from build123d import *

# Parameters (mm, degrees)
SKETCH_W                        = 78
SKETCH_H                        = 68
PAD_DEPTH                       = 29
SKETCH001_W                     = 71
SKETCH001_H                     = 61
POCKET_DEPTH                    = 25
SKETCH002_R                     = 2.5
PAD001_DEPTH                    = 3
SKETCH002_MIRRORED_2_R          = 2.5
PAD001_MIRRORED_2_DEPTH         = 3
SKETCH003_R                     = 3.111428
POCKET001_DEPTH                 = 3
SKETCH004_R                     = 1.4
POCKET002_DEPTH                 = 4
SKETCH004_MIRRORED002_2_R       = 1.4
POCKET002_MIRRORED002_2_DEPTH   = 4
SKETCH005_R                     = 2.5
PAD002_DEPTH                    = 3
SKETCH006_R                     = 1.1
POCKET003_DEPTH                 = 3
SKETCH007_W                     = 9
SKETCH007_H                     = 5
POCKET004_DEPTH                 = 3.5
SKETCH008_W                     = 9
SKETCH008_H                     = 5
POCKET005_DEPTH                 = 3.5
SKETCH009_R                     = 3
POCKET006_DEPTH                 = 3.5
FILLET_R                        = 2
CHAMFER_SIZE                    = 1
CHAMFER001_SIZE                 = 3
SKETCH010_R                     = 2
POCKET007_DEPTH                 = 282.933548
SKETCH010_LINEARPATTERN_2_R     = 2
POCKET007_LINEARPATTERN_2_DEPTH = 282.933548
SKETCH010_LINEARPATTERN_3_R     = 2
POCKET007_LINEARPATTERN_3_DEPTH = 282.933548
SKETCH010_LINEARPATTERN_4_R     = 2
POCKET007_LINEARPATTERN_4_DEPTH = 282.933548
SKETCH010_LINEARPATTERN_5_R     = 2
POCKET007_LINEARPATTERN_5_DEPTH = 282.933548
SKETCH010_LINEARPATTERN_6_R     = 2
POCKET007_LINEARPATTERN_6_DEPTH = 282.933548
SKETCH010_LINEARPATTERN_7_R     = 2
POCKET007_LINEARPATTERN_7_DEPTH = 282.933548
SKETCH010_LINEARPATTERN_8_R     = 2
POCKET007_LINEARPATTERN_8_DEPTH = 282.933548
SKETCH010_LINEARPATTERN_9_R     = 2
POCKET007_LINEARPATTERN_9_DEPTH = 282.933548
LINEARPATTERN001_COUNT          = 3
LINEARPATTERN001_PITCH          = 5
SKETCH011_W                     = 75
SKETCH011_H                     = 65
POCKET008_DEPTH                 = 3
SKETCH012_R                     = 1.564418
PAD003_DEPTH                    = 1


with BuildPart() as part:
    # Sketch → Pad (new body)
    with BuildSketch(Plane.XY):
        with Locations((39, 34)):
            Rectangle(SKETCH_W, SKETCH_H)
    extrude(amount=PAD_DEPTH)

    # Sketch001 (on Face6 of Pad) → Pocket (cut)
    with BuildSketch(Plane.XY.offset(29)):
        with Locations((39, 34)):
            Rectangle(SKETCH001_W, SKETCH001_H)
    extrude(amount=-POCKET_DEPTH, mode=Mode.SUBTRACT)

    # Sketch002 (on Face11 of Pocket) → Pad001 (join)
    with BuildSketch(Plane.XY.offset(4)):
        with Locations((8.5, 60)):
            Circle(SKETCH002_R)
    pad001 = extrude(amount=PAD001_DEPTH)

    # Sketch002 Mirrored 2 → Pad001 Mirrored 2 (add)
    with BuildSketch(Plane(origin=(0, 68, 4), x_dir=(1, 0, 0), z_dir=(0, 0, -1))):
        with Locations((8.5, 60)):
            Circle(SKETCH002_MIRRORED_2_R)
    pad001_mirrored_2 = extrude(amount=-PAD001_MIRRORED_2_DEPTH)

    # Mirrored001: Pad001, Pad001 Mirrored 2 across Sketch002 Axis3
    add(pad001.mirror(Plane(origin=(39, 64.5, 4), x_dir=(0, 0, 1), z_dir=(1, 0, 0))))
    add(pad001_mirrored_2.mirror(Plane(origin=(39, 64.5, 4), x_dir=(0, 0, 1), z_dir=(1, 0, 0))))

    # Sketch003 (on Face17 of MultiTransform) → Pocket001 (cut)
    with BuildSketch(Plane.XY.offset(7)):
        with Locations((69.5, 8)):
            Circle(SKETCH003_R)
    extrude(amount=-POCKET001_DEPTH, mode=Mode.SUBTRACT)

    # Sketch004 (on Face18 of Pocket001) → Pocket002 (cut)
    with BuildSketch(Plane.XY.offset(7)):
        with Locations((8.5, 60)):
            Circle(SKETCH004_R)
    pocket002 = extrude(amount=-POCKET002_DEPTH, mode=Mode.SUBTRACT)

    # Sketch004 Mirrored002 2 → Pocket002 Mirrored002 2 (cut)
    with BuildSketch(Plane(origin=(78, 0, 7), x_dir=(-1, 0, 0), z_dir=(0, 0, -1))):
        with Locations((8.5, 60)):
            Circle(SKETCH004_MIRRORED002_2_R)
    pocket002_mirrored002_2 = extrude(amount=POCKET002_MIRRORED002_2_DEPTH, mode=Mode.SUBTRACT)

    # Mirrored003: Pocket002, Pocket002 Mirrored002 2 across Sketch004 Axis2
    add(pocket002.mirror(Plane(origin=(39, 34, 7), x_dir=(0, 0, 1), z_dir=(0, 1, 0))), mode=Mode.SUBTRACT)
    add(pocket002_mirrored002_2.mirror(Plane(origin=(39, 34, 7), x_dir=(0, 0, 1), z_dir=(0, 1, 0))), mode=Mode.SUBTRACT)

    # Sketch005 (on Face11 of MultiTransform001) → Pad002 (join)
    with BuildSketch(Plane.XY.offset(4)):
        with Locations((49.5, 18)):
            Circle(SKETCH005_R)
    extrude(amount=PAD002_DEPTH)

    # Sketch006 (on Face19 of Pad002) → Pocket003 (cut)
    with BuildSketch(Plane.XY.offset(7)):
        with Locations((69.5, 60)):
            Circle(SKETCH006_R)
    extrude(amount=-POCKET003_DEPTH, mode=Mode.SUBTRACT)

    # Sketch007 (on Face3 of Pocket003) → Pocket004 (cut)
    with BuildSketch(Plane.YZ.offset(78)):
        with Locations((9.9, 11)):
            Rectangle(SKETCH007_W, SKETCH007_H)
    extrude(amount=-POCKET004_DEPTH, mode=Mode.SUBTRACT)

    # Sketch008 (on Face2 of Pocket004) → Pocket005 (cut)
    with BuildSketch(Plane(origin=(0, 0, 0), x_dir=(0, -1, 0), z_dir=(-1, 0, 0))):
        with Locations((-15.4, 11)):
            Rectangle(SKETCH008_W, SKETCH008_H)
    extrude(amount=-POCKET005_DEPTH, mode=Mode.SUBTRACT)

    # Sketch009 (on Face2 of Pocket005) → Pocket006 (cut)
    with BuildSketch(Plane(origin=(0, 0, 0), x_dir=(0, -1, 0), z_dir=(-1, 0, 0))):
        with Locations((-46, 11)):
            Circle(SKETCH009_R)
    extrude(amount=-POCKET006_DEPTH, mode=Mode.SUBTRACT)

    # Fillet
    fillet_edges = [part.edges().sort_by_distance(p)[0] for p in [
        (39, 0, 0),
        (78, 34, 0),
        (39, 68, 0),
        (0, 34, 0),
        (78, 0, 14.5),
        (0, 68, 14.5),
        (78, 68, 14.5),
        (0, 0, 14.5),
    ]]
    fillet(fillet_edges, radius=FILLET_R)

    # Chamfer
    chamfer_edges = [part.edges().sort_by_distance(p)[0] for p in [
        (78, 9.9, 8.5),
        (78, 5.4, 11),
        (78, 9.9, 13.5),
        (78, 14.4, 11),
        (0, 15.4, 8.5),
        (0, 19.9, 11),
        (0, 15.4, 13.5),
        (0, 10.9, 11),
    ]]
    chamfer(chamfer_edges, length=CHAMFER_SIZE)

    # Chamfer001
    chamfer001_edges = [part.edges().sort_by_distance(p)[0] for p in [
        (0, 49, 11),
    ]]
    chamfer(chamfer001_edges, length=CHAMFER001_SIZE)

    # Sketch010 (on Face16 of Chamfer001) → Pocket007 (cut, through all)
    with BuildSketch(Plane.XZ):
        with Locations((7, 12.5)):
            Circle(SKETCH010_R)
    pocket007 = extrude(amount=-POCKET007_DEPTH, mode=Mode.SUBTRACT)

    # Sketch010 LinearPattern 2 → Pocket007 LinearPattern 2 (cut, through all)
    with BuildSketch(Plane(origin=(8, 0, 0), x_dir=(1, 0, 0), z_dir=(0, -1, 0))):
        with Locations((7, 12.5)):
            Circle(SKETCH010_LINEARPATTERN_2_R)
    pocket007_linearpattern_2 = extrude(amount=-POCKET007_LINEARPATTERN_2_DEPTH, mode=Mode.SUBTRACT)

    # Sketch010 LinearPattern 3 → Pocket007 LinearPattern 3 (cut, through all)
    with BuildSketch(Plane(origin=(16, 0, 0), x_dir=(1, 0, 0), z_dir=(0, -1, 0))):
        with Locations((7, 12.5)):
            Circle(SKETCH010_LINEARPATTERN_3_R)
    pocket007_linearpattern_3 = extrude(amount=-POCKET007_LINEARPATTERN_3_DEPTH, mode=Mode.SUBTRACT)

    # Sketch010 LinearPattern 4 → Pocket007 LinearPattern 4 (cut, through all)
    with BuildSketch(Plane(origin=(24, 0, 0), x_dir=(1, 0, 0), z_dir=(0, -1, 0))):
        with Locations((7, 12.5)):
            Circle(SKETCH010_LINEARPATTERN_4_R)
    pocket007_linearpattern_4 = extrude(amount=-POCKET007_LINEARPATTERN_4_DEPTH, mode=Mode.SUBTRACT)

    # Sketch010 LinearPattern 5 → Pocket007 LinearPattern 5 (cut, through all)
    with BuildSketch(Plane(origin=(32, 0, 0), x_dir=(1, 0, 0), z_dir=(0, -1, 0))):
        with Locations((7, 12.5)):
            Circle(SKETCH010_LINEARPATTERN_5_R)
    pocket007_linearpattern_5 = extrude(amount=-POCKET007_LINEARPATTERN_5_DEPTH, mode=Mode.SUBTRACT)

    # Sketch010 LinearPattern 6 → Pocket007 LinearPattern 6 (cut, through all)
    with BuildSketch(Plane(origin=(40, 0, 0), x_dir=(1, 0, 0), z_dir=(0, -1, 0))):
        with Locations((7, 12.5)):
            Circle(SKETCH010_LINEARPATTERN_6_R)
    pocket007_linearpattern_6 = extrude(amount=-POCKET007_LINEARPATTERN_6_DEPTH, mode=Mode.SUBTRACT)

    # Sketch010 LinearPattern 7 → Pocket007 LinearPattern 7 (cut, through all)
    with BuildSketch(Plane(origin=(48, 0, 0), x_dir=(1, 0, 0), z_dir=(0, -1, 0))):
        with Locations((7, 12.5)):
            Circle(SKETCH010_LINEARPATTERN_7_R)
    pocket007_linearpattern_7 = extrude(amount=-POCKET007_LINEARPATTERN_7_DEPTH, mode=Mode.SUBTRACT)

    # Sketch010 LinearPattern 8 → Pocket007 LinearPattern 8 (cut, through all)
    with BuildSketch(Plane(origin=(56, 0, 0), x_dir=(1, 0, 0), z_dir=(0, -1, 0))):
        with Locations((7, 12.5)):
            Circle(SKETCH010_LINEARPATTERN_8_R)
    pocket007_linearpattern_8 = extrude(amount=-POCKET007_LINEARPATTERN_8_DEPTH, mode=Mode.SUBTRACT)

    # Sketch010 LinearPattern 9 → Pocket007 LinearPattern 9 (cut, through all)
    with BuildSketch(Plane(origin=(64, 0, 0), x_dir=(1, 0, 0), z_dir=(0, -1, 0))):
        with Locations((7, 12.5)):
            Circle(SKETCH010_LINEARPATTERN_9_R)
    pocket007_linearpattern_9 = extrude(amount=-POCKET007_LINEARPATTERN_9_DEPTH, mode=Mode.SUBTRACT)

    # LinearPattern001: Pocket007, Pocket007 LinearPattern 2, Pocket007 LinearPattern 3, Pocket007 LinearPattern 4, Pocket007 LinearPattern 5, Pocket007 LinearPattern 6, Pocket007 LinearPattern 7, Pocket007 LinearPattern 8, Pocket007 LinearPattern 9 ×3
    with Locations(*[(0, 0, i * LINEARPATTERN001_PITCH) for i in range(1, LINEARPATTERN001_COUNT)]):
        add(pocket007, mode=Mode.SUBTRACT)
        add(pocket007_linearpattern_2, mode=Mode.SUBTRACT)
        add(pocket007_linearpattern_3, mode=Mode.SUBTRACT)
        add(pocket007_linearpattern_4, mode=Mode.SUBTRACT)
        add(pocket007_linearpattern_5, mode=Mode.SUBTRACT)
        add(pocket007_linearpattern_6, mode=Mode.SUBTRACT)
        add(pocket007_linearpattern_7, mode=Mode.SUBTRACT)
        add(pocket007_linearpattern_8, mode=Mode.SUBTRACT)
        add(pocket007_linearpattern_9, mode=Mode.SUBTRACT)

    # Sketch011 (on Face7 of MultiTransform002) → Pocket008 (cut)
    with BuildSketch(Plane.XY.offset(29)):
        with Locations((39, 34)):
            Rectangle(SKETCH011_W, SKETCH011_H)
    extrude(amount=-POCKET008_DEPTH, mode=Mode.SUBTRACT)

    # Sketch012 (on Face117 of Pocket008) → Pad003 (join)
    with BuildSketch(Plane.XY.offset(3)):
        with Locations((69.449699, 7.994386)):
            Circle(SKETCH012_R)
    extrude(amount=PAD003_DEPTH)


solid = part.part
Part model, mm, in its own coordinate system. A direction names the side the tool comes from. Give positions to 0.01 mm unless a question says otherwise; leave off trailing zeros. Loops run counter-clockwise (first coordinate to the right, second up) from the corner with the lowest first, then second, coordinate; pieces in that order, holes last. Notation, with made-up numbers: M 80.5,20 L 100.5,20 A19 ccw 100.5,27 Z; hole C 44.5,37.5 d1. An arc over 180 degrees is marked long. Put each result on its own line as item: value. Start each with the question number.
1) Saw through at C-C (x = 43.5). List the corners of the cut face in (y, z).
2) Flat gauge pins, fed straight in: pin 1 (2 mm diameter, centred on x = 8.5, y = 60.5, fed in from +Z); pin 2 (0.8 mm diameter, centred on x = 2, y = 14.5, fed in from +Z); pin 3 (3 mm diameter, centred on x = 40.5, y = 39.5, fed in from +Z). Where does each tip first touch, or does it go through?
3) 3-axis set-ups, long thin cutter, end or side, ignore diameter. For faces 1 (the cylindrical face through (71, 58, 5)), 2 (the flat face through (2, 15, 13.5)), 3 (the cylindrical face through (21.4, 1.7, 21.3)): which of +Z, -Z, +X, -X, +Y, -Y reach the whole face in a straight line?
4) Saw through at D-D (y = 46). List the corners of the cut face in (x, z).
5) Saw through at B-B (y = 29). List the corners of the cut face in (x, z), then the cut area to 3 significant figures.
6) Pull direction Z, two halves, no side cores. Call faces 4 (the cylindrical face through (0.57, 34.45, 0.6)), 5 (the flat face through (8, 8, 3)), 6 (the flat face through (2, 10.9, 11)): +Z half, -Z half, draft (parallel to the pull), parting line (faces both ways), or undercut.
7) Saw through at A-A (y = 8). List the corners of the cut face in (x, z).
8) Probe probe 1 along Z at (x, y) = (15, 2.85); probe 2 along Y at (x, z) = (22.5, 9.5); probe 3 along X at (y, z) = (54, 8). List the from-to ranges inside material, lowest first.
Numbers:
1. outline: M 0,2 A2 ccw 2,0 L 66,0 A2 ccw 68,2 L 68,29 L 66.5,29 L 66.5,26 L 64.5,26 L 64.5,4 L 3.5,4 L 3.5,26 L 1.5,26 L 1.5,29 L 0,29 Z
2. pin 1: z = 7
2. pin 2: z = 26
2. pin 3: z = 4
3. face 1: +Z
3. face 2: -X
3. face 3: +Y, -Y
4. outline: M 0,2 A2 ccw 2,0 L 76,0 A2 ccw 78,2 L 78,29 L 76.5,29 L 76.5,26 L 74.5,26 L 74.5,4 L 3.5,4 L 3.5,8 L 3,8 L 0,5 Z; M 0,17 L 3,14 L 3.5,14 L 3.5,26 L 1.5,26 L 1.5,29 L 0,29 Z
5. outline: M 0,2 A2 ccw 2,0 L 76,0 A2 ccw 78,2 L 78,29 L 76.5,29 L 76.5,26 L 74.5,26 L 74.5,4 L 3.5,4 L 3.5,26 L 1.5,26 L 1.5,29 L 0,29 Z
5. area: 473 mm^2
6. face 4: -Z half
6. face 5: +Z half
6. face 6: undercut
7. outline: M 0,2 A2 ccw 2,0 L 76,0 A2 ccw 78,2 L 78,7.5 L 77,8.5 L 74.5,8.5 L 74.5,4 L 11,4 L 11,7 L 9.9,7 L 9.9,3 L 7.1,3 L 7.1,7 L 6,7 L 6,4 L 3.5,4 L 3.5,26 L 1.5,26 L 1.5,29 L 0,29 Z; M 74.5,13.5 L 77,13.5 L 78,14.5 L 78,29 L 76.5,29 L 76.5,26 L 74.5,26 Z
8. probe 1: 0 to 10.5, 14.5 to 15.5, 19.5 to 20.5, 24.5 to 26
8. probe 2: 0 to 3.5, 64.5 to 68
8. probe 3: 0 to 3.5, 74.5 to 78
